Autodesk Inventor part; units mm, degrees
ref_plane "Work Plane1" through (0, 0, -15) normal (0, 0, 1) x (1, 0, 0)
ref_plane "YZ Plane" through (0, 0, 0) normal (1, 0, 0) x (0, 1, 0)
ref_plane "XZ Plane" through (0, 0, 0) normal (0, 1, 0) x (-1, 0, 0)
sketch "Sketch1" plane through (0, 0, 0) normal (0, 0, 1) x (1, 0, 0)
  line L0 (0, 0) -> (25, 0)
  line L1 (25, 0) -> (25, 40)
  line L2 (25, 40) -> (0, 40)
  line L3 (0, 40) -> (0, 0)
  dimension "d1" = 25
  dimension "d2" = 40
  dimension "d3" = 25
extrude "Extrusion1" add sketch "Sketch1" against normal blind 30
sketch "Sketch2" plane through (25, 0, 0) normal (1, 0, 0) x (0, 0, -1)
  line L0 (0, 0) -> (30, 0)
  circle A0 centre (15, 6.56) radius 2.46
extrude "Extrusion2" cut sketch "Sketch2" against normal blind 30
sketch "Sketch3" plane through (0, 0, 0) normal (-1, 0, 0) x (0, 0, 1)
  line L0 (0, 0) -> (-30, 0)
  line L1 (-25.05, 0) -> (-4.95, 0)
  line L2 (-4.95, 0) -> (-4.95, 33.12)
  line L3 (-4.95, 33.12) -> (-25.05, 33.12)
  line L4 (-25.05, 33.12) -> (-25.05, 0)
  dimension "d11" = 20.1
extrude "Extrusion3" cut sketch "Sketch3" against normal blind 20
sketch "Sketch4" plane through (0, 0, 0) normal (0, -1, 0) x (1, 0, 0)
  line L0 (20, -4.95) -> (20, -25.05)
  line L1 (20, -15) -> (25, -15)
  line L2 (25, 0) -> (25, -30)
  line L3 (20, -8.025) -> (25, -8.025)
  line L4 (25, -8.025) -> (25, -21.975)
  line L5 (25, -21.975) -> (20, -21.975)
  line L6 (20, -21.975) -> (20, -8.025)
  line L7 (20, -8.025) -> (25, -21.975) construction
  line L8 (25, -8.025) -> (20, -21.975) construction
  line L9 (25, -12.54) -> (25, -17.46)
  point P0 (0, 0)
  point P1 (22.5, -15)
  dimension "d14" = 13.95
extrude "Extrusion4" add sketch "Sketch4" along normal blind 15
sketch "Sketch5" plane through (20, 0, 0) normal (-1, 0, 0) x (0, 0, 1)
  circle A0 centre (-15, 6.56) radius 2.46
  circle A1 centre (-15, 6.56) radius 4.7025
  circle A2 centre (-15, 6.56) radius 2.46
  circle A3 centre (-15, 6.56) radius 2.46
  point P0 (0, 0)
  dimension "d17" = 9.405
extrude "Extrusion5" cut sketch "Sketch5" against normal blind 2.1
sketch "Sketch6" plane through (25, 0, 0) normal (1, 0, 0) x (0, 0, -1)
  circle A0 centre (15, 6.56) radius 4.7025
  line L0 (15, 6.56) -> (15, 23.56)
  circle A1 centre (15, 23.56) radius 2.46
  point P0 (0, 0)
  dimension "d20" = 17
  dimension "d21" = 4.92
extrude "Extrusion6" cut sketch "Sketch6" against normal blind 10 contours A1
sketch "Sketch7" plane through (20, 0, 0) normal (-1, 0, 0) x (0, 0, 1)
  circle A0 centre (-15, 23.56) radius 2.46
  circle A1 centre (-15, 23.56) radius 4.7025
  point P0 (0, 0)
  dimension "d24" = 9.405
extrude "Extrusion7" cut sketch "Sketch7" against normal blind 2.1
sketch "Sketch9" plane through (25, 0, 0) normal (1, 0, 0) x (0, 0, -1)
  circle A0 centre (15, 6.56) radius 2.46
  circle A1 centre (15, 6.56) radius 2.46
  circle A2 centre (15, 23.56) radius 2.46
  circle A3 centre (15, 23.56) radius 2.46
  line L0 (30, 40) -> (30, 0)
  line L1 (30, 0) -> (30, 40)
  line L2 (30, 40) -> (0, 40)
  line L3 (0, 40) -> (0, 0)
  line L4 (0, 0) -> (8.025, 0)
  line L5 (21.975, 0) -> (21.975, -15)
  line L6 (21.975, -15) -> (8.025, -15)
  line L7 (8.025, -15) -> (8.025, 0)
  line L8 (0, 0) -> (8.025, 0)
  line L9 (21.975, 0) -> (30, 0)
extrude "Extrusion8" add sketch "Sketch9" along normal blind 5
sketch "Sketch10" plane through (0, 40, 0) normal (0, 1, 0) x (1, 0, 0)
  line L0 (0, 30) -> (30, 30)
  line L1 (30, 0) -> (0, 0)
  line L2 (0, 30) -> (30, 30)
  line L3 (30, 30) -> (30, 0)
  line L4 (30, 0) -> (0, 0)
  line L5 (0, 0) -> (0, 30)
extrude "Extrusion9" add sketch "Sketch10" along normal blind 30
sketch "Sketch12" plane through (30, 0, 0) normal (1, 0, 0) x (0, 0, -1)
  circle A0 centre (15, 6.56) radius 2.46
  line L0 (15, 6.56) -> (15, 15.06)
  circle A1 centre (15, 15.06) radius 2.525
  point P0 (0, 0)
  dimension "d31" = 8.5
  dimension "d33" = 5.05
extrude "Extrusion10" cut sketch "Sketch12" against normal blind 30 contours A1
sketch "Sketch14" plane through (0, 0, 0) normal (0, 0, 1) x (1, 0, 0)
  line L0 (30, 70) -> (0, 70)
  line L1 (0, 70) -> (0, 85)
  line L2 (-15, 100) -> (-23, 100)
  line L3 (30, 100) -> (15, 115)
  line L4 (-23, 115) -> (15, 115)
  line L5 (30, 0) -> (30, 70)
  line L6 (30, 100) -> (30, 70)
  line L7 (-20.5, 113.5) -> (-23, 115)
  line L8 (-20.5, 101.5) -> (-23, 100)
  line L9 (-18, 107.5) -> (-20.5, 101.5)
  line L10 (-18, 107.5) -> (-20.5, 113.5)
  arc A0 (0, 85) -> (-15, 100) centre (-15, 85) ccw
  point P0 (0, 0)
  point P1 (0, 100)
  dimension "d47" = 30
  dimension "d49" = 15
  dimension "d54" = 15
extrude "Extrusion12" add sketch "Sketch14" against normal blind 30
sketch "Sketch15" plane through (0, 0, -25.05) normal (-1, 0, 0) x (0, 0, 1)
  line L0 (0, 33.12) -> (20.1, 33.12)
  line L1 (20.1, 33.12) -> (20.1, 0)
  line L2 (0, 33.12) -> (20.1, 33.12)
  line L3 (20.1, 33.12) -> (20.1, 31.1)
  line L4 (20.1, 31.1) -> (0, 31.1)
  line L5 (0, 31.1) -> (0, 33.12)
  point P0 (25.05, 0)
  dimension "d57" = 2.02
extrude "Extrusion13" add sketch "Sketch15" against normal blind 20
sketch "Sketch17" plane through (0, 0, 0) normal (0, 0, 1) x (1, 0, 0)
  line L0 (-23, 115) -> (15, 115)
  line L1 (-23, 115) -> (15, 115)
  line L2 (30, 0) -> (30, 100)
  line L3 (15, 115) -> (30, 100)
  line L4 (30, 100) -> (30, 85)
  arc A0 (0, 85) -> (-15, 100) centre (-15, 85) ccw
  line L5 (30, 85) -> (0, 85)
  arc A1 (0, 85) -> (-15, 100) centre (-15, 85) ccw
  line L6 (-15, 100) -> (-23, 100)
  line L7 (-15, 100) -> (-23, 100)
  line L8 (-23, 100) -> (-20.5, 101.5)
  line L9 (-23, 100) -> (-20.5, 101.5)
  line L10 (-20.5, 101.5) -> (-18, 107.5)
  line L11 (-20.5, 101.5) -> (-18, 107.5)
  line L12 (-18, 107.5) -> (-20.5, 113.5)
  line L13 (-18, 107.5) -> (-20.5, 113.5)
  line L14 (-20.5, 113.5) -> (-23, 115)
  point P0 (0, 0)
extrude "Extrusion14" add sketch "Sketch17" along normal blind 30
ref_plane "Work Plane1" through (0, 0, -15) normal (0, 0, 1) x (1, 0, 0)
mirror "Mirror1" about plane through (0, 0, -15) normal (0, 0, 1) of "Extrusion14"
properties part number "12mm_x_90mm"
Geometry: final body of the model. Coordinates: model frame, mm. A direction names the side the tool comes from. Give positions to 0.01 mm unless a question says otherwise; leave off trailing zeros. Write each loop counter-clockwise with the first axis right and the second up, starting at its lowest first coordinate (ties: lowest second). Pieces come first, ordered by that corner, then holes.
(1) Access query for faces 4 (the flat face through (-19.232, 104.542, -14.37)), 5 (the flat face through (18, 0, -27)), 6 (the flat face through (22.1, 4.5, -13)). Directions: +Z, -Z, +X, -X, +Y, -Y. A direction counts if a zero-diameter tool reaches every point of the face in a straight line with its end or side. Return the directions, or none.
(2) Cut plane D-D, the plane x = 4.5. Return loops of the section in (y, z).
(3) Cut plane C-C, the plane x = 24. Return loops of the section in (y, z) (3 decimals).
(4) Cut plane B-B, the plane y = 23.56. Return loops of the section in (x, z), then the cut area to 3 significant figures.
(5) Mould query, pull axis Y, two halves, no side actions, for faces 1 (the cylindrical face through (25.07, 15.171, -12.477)), 2 (the flat face through (15, 0, -3)), 3 (the flat face through (20, 8, -20)). Classes: released by +Y, released by -Y, zero draft, split by the parting line, or undercut.
(6) First-contact query: P1, Ø24, axis at y = 61, z = -8.5, coming from the -X side; P2, Ø2, axis at x = 18.5, y = 58, coming from the -Z side; P3, Ø24, axis at x = 17, y = 52.5, coming from the +Z side; P4, Ø4.5, axis at y = 15.06, z = -15, coming from the +X side. Flat tips, straight axial feed; report the tip coordinate or a pass-through.
(7) Cut plane A-A, the plane z = -15. Give the number of separate pieces and of enclosed holes in the cut face, then the cut area to 3 significant figures.
(8) Ray query, line 1 (Z direction, x = 26, y = 6.56); line 2 (Y direction, x = 25.5, z = -15) (3 decimals); line 3 (Y direction, x = 26, z = -15) (3 decimals). Return the intervals inside material, ascending.
Values follow:
1. face 4: +Z, -Z, -X
1. face 5: -Z, +X, -X, -Y
1. face 6: -X
2. outline: (0, -30) - (85, -30) - (85, -60) - (115, -60) - (115, 30) - (85, 30) - (85, 0) - (0, 0) - (0, -4.95) - (31.1, -4.95) - (31.1, -25.05) - (0, -25.05) - close
3. outline: (-15, -21.975) - (0, -21.975) - (0, -30) - (85, -30) - (85, -60) - (106, -60) - (106, 30) - (85, 30) - (85, 0) - (0, 0) - (0, -8.025) - (-15, -8.025) - close; hole circle Ø4.92 at (6.56, -15); hole circle Ø5.05 at (15.06, -15); hole circle Ø4.92 at (23.56, -15)
4. outline: (0, -30) - (30, -30) - (30, -17.46) - (22.1, -17.46) - (22.1, -19.7) - (20, -19.7) - (20, -25.05) - (0, -25.05) - close; (0, -4.95) - (20, -4.95) - (20, -10.3) - (22.1, -10.3) - (22.1, -12.54) - (30, -12.54) - (30, 0) - (0, 0) - close
4. area: 439 mm2
5. face 1: undercut
5. face 2: released by -Y
5. face 3: zero draft
6. P1: stops at x = 0
6. P2: stops at z = -30
6. P3: stops at z = 0
6. P4: passes through
7. separate pieces: 4
7. enclosed holes: 0
7. area: 3,040 mm2
8. line 1: z = -30 to -17.46, -12.54 to 0
8. line 2: y = -15 to 4.1, 9.02 to 12.535, 17.585 to 21.1, 26.02 to 104.5
8. line 3: y = -15 to 4.1, 9.02 to 12.535, 17.585 to 21.1, 26.02 to 104
